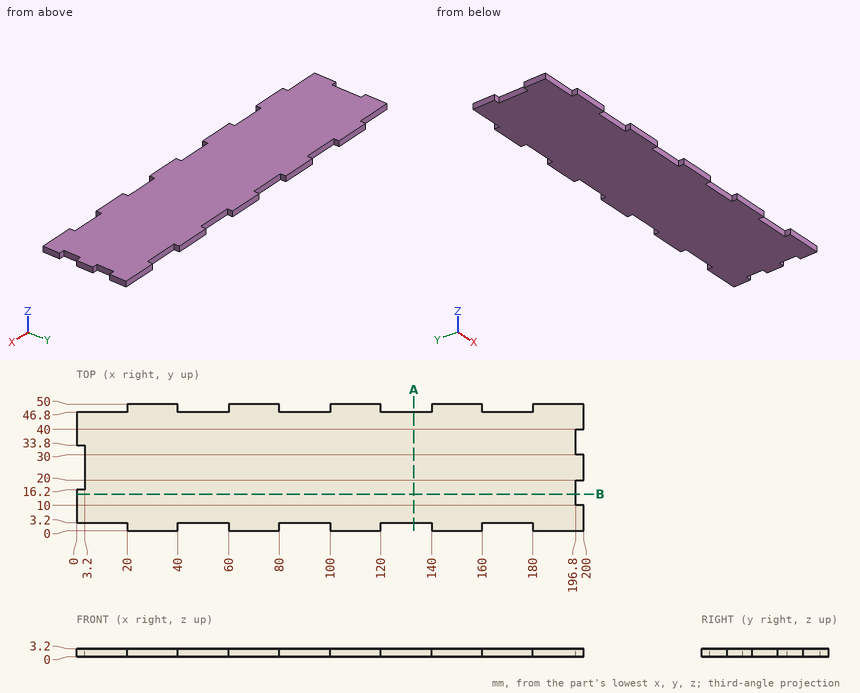
Design review of the part shown in the three views and the two pictorial views. Dimensions are in mm from the part's minimum x, y and z. Round coordinates to 2 decimals unless told otherwise and drop trailing zeros. Loops run counter-clockwise (first coordinate to the right, second up) from the corner with the lowest first, then second, coordinate; pieces in that order, holes last. Notation, with made-up numbers: M 83,19.5 L 91,19.5 A13 cw 91,23.5 Z; hole C 3,7.25 d7. An arc over 180 degrees is marked long. Put each result on its own line as item: value.
Q1. Consider section A-A, the plane x = 133. Give the boundary of the cut face in (y, z).
Result set:
outline: M 3.2,0 L 46.8,0 L 46.8,3.2 L 3.2,3.2 Z
Q2. Consider section B-B, the plane y = 14.5. Give the boundary of the cut face in (x, z), then the cut area to 3 significant figures.
Result set:
outline: M 0,0 L 196.8,0 L 196.8,3.2 L 0,3.2 Z
area: 630 mm²
Q3. To check wall thickness, follow L1, parallel to X at y = 47, z = 0.55; L2, parallel to X at y = 15.5, z = 2.3; L3, parallel to X at y = 25, z = 2.3. State the ranges of each line that lie inside material, in increasing order.
Result set:
L1: x = 20 to 40, 60 to 80, 100 to 120, 140 to 160, 180 to 200
L2: x = 0 to 196.8
L3: x = 3.2 to 200
Q4. For pin 1 (1 mm diameter, centred on x = 175, z = 1.5, fed in from +Y); pin 2 (1.6 mm diameter, centred on x = 86.5, z = 1.5, fed in from -Y); pin 3 (1.6 mm diameter, centred on y = 2.5, z = 1, fed in from -X); pin 4 (1 mm diameter, centred on y = 39, z = 1, fed in from +X), all flat-tipped, find the tip position at first contact; note any pin that passes through.
Result set:
pin 1: stops at y = 46.8
pin 2: stops at y = 3.2
pin 3: stops at x = 0
pin 4: stops at x = 196.8
